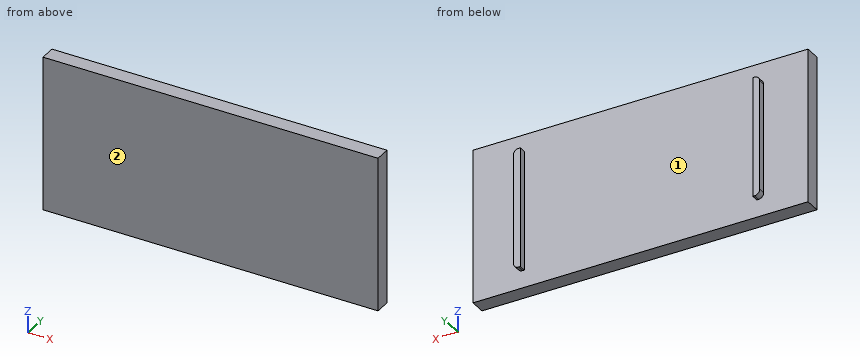
from build123d import *

# Parameters (mm, degrees)
ESQUISSE1_W                 = 160
ESQUISSE1_H                 = 90
T_LE_DE_BASE_PLI_E1_DEPTH   = 9
T_LE_PLI_E_SUR_AR_TE1_DEPTH = 90
T_LE_PLI_E_SUR_AR_TE2_DEPTH = 90
EXTRUSION1_DEPTH            = 4
ETAT_START                  = -116.640587823
ETAT_D_PLI_1_OUTLINE_W      = 10
ETAT_D_PLI_1_OUTLINE_H      = 90
ETAT_D_PLI_1_DEPTH          = 179.4732
ETAT_START_2                = -124.393019868
ETAT_D_PLI_1_2_OUTLINE_W    = 9
ETAT_D_PLI_1_2_OUTLINE_H    = 90
ETAT_D_PLI_1_2_DEPTH        = 194.978064089
ECHELLE1_SCALE              = 1.07


# Read off the part's stored shape, not the designer's step: Etat déplié1
# Sheet-metal steps are written as plain solids
with BuildPart() as part:
    # Esquisse1 → Tôle de base pliée1 (new body)
    with BuildSketch(Plane(origin=(0, 0, 0), x_dir=(1, 0, 0), z_dir=(0, 1, 0))):
        with Locations((-26.903987823, 16.826605784)):
            Rectangle(ESQUISSE1_W, ESQUISSE1_H)
    extrude(amount=T_LE_DE_BASE_PLI_E1_DEPTH)

    # Tôle pliée sur arête1 section (across the edge) → Tôle pliée sur arête1 (add)
    with BuildSketch(Plane(origin=(53.832612177, 0, -61.826605784), x_dir=(-1, 0, 0), z_dir=(0, 0, 1))):
        with BuildLine():
            Line((-9, 0.7366), (-9, 10))
            Line((-9, 10), (0, 10))
            Line((0, 10), (0, 0.7366))
            ThreePointArc((0, 0.7366), (0.215745145, 0.215745145), (0.7366, 0))
            Line((0.7366, 0), (0.7366, -9))
            ThreePointArc((0.7366, -9), (-6.148215886, -6.148215886), (-9, 0.7366))
        make_face()
    extrude(amount=T_LE_PLI_E_SUR_AR_TE1_DEPTH)

    # Tôle pliée sur arête2 section (across the edge) → Tôle pliée sur arête2 (add)
    with BuildSketch(Plane(origin=(-107.640587823, 0, 28.173394216), x_dir=(1, 0, 0), z_dir=(0, 0, -1))):
        with BuildLine():
            Line((-9, 0.7366), (-9, 10))
            Line((-9, 10), (0, 10))
            Line((0, 10), (0, 0.7366))
            ThreePointArc((0, 0.7366), (0.215745145, 0.215745145), (0.7366, 0))
            Line((0.7366, 0), (0.7366, -9))
            ThreePointArc((0.7366, -9), (-6.148215886, -6.148215886), (-9, 0.7366))
        make_face()
    extrude(amount=T_LE_PLI_E_SUR_AR_TE2_DEPTH)

    # Esquisse9 → Extrusion1 (add)
    with BuildSketch(Plane(origin=(0, 9, 0), x_dir=(1, 0, 0), z_dir=(0, 1, 0))):
        with BuildLine():
            Line((-95.557213934, 51.644704016), (-94.557213934, 51.644704016))
            Line((-94.557213934, 51.644704016), (-94.557213934, -18.355295984))
            Line((-94.557213934, -18.355295984), (-95.557213934, -18.355295984))
            ThreePointArc((-95.557213934, -18.355295984), (-97.678534277, -17.476616327), (-98.557213934, -15.355295984))
            Line((-98.557213934, -15.355295984), (-98.557213934, 48.644704016))
            ThreePointArc((-98.557213934, 48.644704016), (-97.678534277, 50.76602436), (-95.557213934, 51.644704016))
        make_face()
        with BuildLine():
            Line((40.749238287, 51.644704016), (40.749238287, -18.355295984))
            Line((40.749238287, -18.355295984), (41.749238287, -18.355295984))
            ThreePointArc((41.749238287, -18.355295984), (43.870558631, -17.476616327), (44.749238287, -15.355295984))
            Line((44.749238287, -15.355295984), (44.749238287, 48.644704016))
            ThreePointArc((44.749238287, 48.644704016), (43.870558631, 50.76602436), (41.749238287, 51.644704016))
            Line((41.749238287, 51.644704016), (40.749238287, 51.644704016))
        make_face()
    extrude(amount=EXTRUSION1_DEPTH)

    # Etat déplié1 outline → Etat déplié1 (cut)
    with BuildSketch(Plane.YZ.offset(ETAT_START)):
        with Locations((-5, -16.826605784)):
            Rectangle(ETAT_D_PLI_1_OUTLINE_W, ETAT_D_PLI_1_OUTLINE_H)
    extrude(amount=ETAT_D_PLI_1_DEPTH, mode=Mode.SUBTRACT)

    # Etat d_pli_1 2 outline → Etat d_pli_1 2 (add)
    with BuildSketch(Plane.YZ.offset(ETAT_START_2)):
        with Locations((4.5, -16.826605784)):
            Rectangle(ETAT_D_PLI_1_2_OUTLINE_W, ETAT_D_PLI_1_2_OUTLINE_H)
    extrude(amount=ETAT_D_PLI_1_2_DEPTH)


with BuildPart() as part_1:
    # Echelle1: scaled about (-26.903987823, 4.589665377, -16.824096508)
    add(part.part.scale(ECHELLE1_SCALE).moved(Location((1.883279148, -0.321276576, 1.177686756))))


solid = part_1.part
Design review of the part built by this model. Coordinates are the model's own, in mm. Face numbers are marked on the shaded views. Give positions to 0.01 mm unless a question says otherwise; leave off trailing zeros. Loops run counter-clockwise (first coordinate to the right, second up) from the corner with the lowest first, then second, coordinate; pieces in that order, holes last. Notation, with made-up numbers: M 27,-36 L 68,-36 A28 ccw 68,-7 Z; hole C 36.5,29.5 d7. An arc over 180 degrees is marked long. One line per question, with ' | ' between items. Start each with the question number.
1. To check wall thickness, follow L1, parallel to Y at x = 56.5, z = -25.5; L2, parallel to Z at x = 47.5, y = 12; L3, parallel to Z at x = -101, y = 12. State the ranges of each line that lie inside material, in increasing order.
2. Add section B-B (z = -42). Write out the cut boundary in (x, y).
3. Add section C-C (x = 33.5). Write out the cut boundary in (y, z), plus the area to 3 significant figures.
4. The part is to be moulded in two halves that separate along X. For the marked faces 1 and 2, say which applies: released by +X, released by -X, zero draft, split by the parting line, or undercut.
5. Insertion check: P1, Ø1.3, axis at y = 11.5, z = -8.5, coming from the +X side; P2, Ø0.5, axis at x = 46, y = 11.5, coming from the +Z side; P3, Ø0.9, axis at x = 46, y = 12.5, coming from the -Z side. Each pin has a flat end and moves straight along its axis. Give the tip position at first contact, or say it passes through.
6. Add section D-D (z = -58.5). Write out the cut boundary in (x, y), plus the area to 3 significant figures.
7. Add section A-A (y = 11.5). Write out the cut boundary in (x, z), plus the area to 3 significant figures.
Worked out:
1) L1: y = -0.32 to 9.31 | L2: z = -53.94 to 20.68 | L3: z = -54.02 to 20.75
2) outline: M -131.22,-0.32 L 77.41,-0.32 L 77.41,9.31 L 49.76,9.31 L 49.76,13.59 L 45.48,13.59 L 45.48,9.31 L -99.29,9.31 L -99.29,13.59 L -103.57,13.59 L -103.57,9.31 L -131.22,9.31 Z
3) outline: M -0.32,-64.98 L 9.31,-64.98 L 9.31,31.32 L -0.32,31.32 Z | area: 927 mm²
4) face 1: undercut | face 2: zero draft
5) P1: stops at x = 49.76 | P2: stops at z = 20.82 | P3: stops at z = -54.08
6) outline: M -131.22,-0.32 L 77.41,-0.32 L 77.41,9.31 L -131.22,9.31 Z | area: 2,010 mm²
7) outline: M -103.57,-50.87 A3.21 ccw -100.36,-54.08 L -99.29,-54.08 L -99.29,20.82 L -100.36,20.82 A3.21 ccw -103.57,17.61 Z; M 45.48,-54.08 L 46.55,-54.08 A3.21 ccw 49.76,-50.87 L 49.76,17.61 A3.21 ccw 46.55,20.82 L 45.48,20.82 Z | area: 632 mm²
